from build123d import *

# Parameters (mm, degrees)
SKETCH1_R           = 250
SKETCH1_R_2         = 162.5
BOSS_EXTRUDE1_DEPTH = 9.5
SKETCH2_R           = 202.5
SKETCH2_R_2         = 192.5
CUT_EXTRUDE1_DEPTH  = 7


with BuildPart() as part:
    # Sketch1 → Boss-Extrude1 (new, symmetric)
    with BuildSketch(Plane(origin=(0, 0, 0), x_dir=(1, 0, 0), z_dir=(0, 1, 0))):
        with Locations(Location((0, 0, 0), (0, 0, 270))):
            Circle(SKETCH1_R)
        with Locations(Location((0, 0, 0), (0, 0, 270))):
            Circle(SKETCH1_R_2, mode=Mode.SUBTRACT)
    extrude(amount=BOSS_EXTRUDE1_DEPTH, both=True)

    # Sketch2 → Cut-Extrude1 (cut)
    with BuildSketch(Plane(origin=(0, 9.5, 0), x_dir=(1, 0, 0), z_dir=(0, 1, 0))):
        with Locations(Location((0, 0, 0), (0, 0, 270))):
            Circle(SKETCH2_R)
        with Locations(Location((0, 0, 0), (0, 0, 270))):
            Circle(SKETCH2_R_2, mode=Mode.SUBTRACT)
    extrude(amount=-CUT_EXTRUDE1_DEPTH, mode=Mode.SUBTRACT)


solid = part.part
CAD build for the part. Positions are in the model's coordinates, mm. A direction names the side the tool comes from. Round coordinates to 2 decimals unless told otherwise and drop trailing zeros. Order: outer loops, then holes, each group sorted by start corner. A loop starts at its lowest first (then second) coordinate and runs counter-clockwise, first axis right, second up. Notation, with made-up numbers: (89.5, 71) -> (108.5, 71) arc R11 ccw to (108.5, 89) -> close; hole circle Ø6 at (38, 66.5). An arc over 180 degrees is marked (long way). Write each question's results on one line, items separated by ' | '.
1. Cut at B-B (x = 0). Give the cut face in (y, z), plus the area to 4 significant figures.
Findings below:
outline: (-9.5, -250) -> (9.5, -250) -> (9.5, -202.5) -> (2.5, -202.5) -> (2.5, -192.5) -> (9.5, -192.5) -> (9.5, -162.5) -> (-9.5, -162.5) -> close; (-9.5, 162.5) -> (9.5, 162.5) -> (9.5, 192.5) -> (2.5, 192.5) -> (2.5, 202.5) -> (9.5, 202.5) -> (9.5, 250) -> (-9.5, 250) -> close | area: 3,185 mm²
2. 3-axis set-ups, long thin cutter, end or side, ignore diameter. For faces 1 (the face through (1, 9.5, 203)), 2 (the face through (-74, 2.5, 179)): which of +Z, -Z, +X, -X, +Y, -Y reach the whole face in a straight line?
Findings below:
face 1: +Z, -Z, +X, -X, +Y | face 2: +Y
3. Cut at D-D (x = 215.5). Give the cut face in (y, z).
Findings below:
outline: (-9.5, -126.73) -> (9.5, -126.73) -> (9.5, 126.73) -> (-9.5, 126.73) -> close
4. Pull direction X, two halves, no side cores. Call faces 3 (the face through (10.99, 0.13, -249.76)), 4 (the face through (137.02, -0.13, 87.36)), 5 (the face through (3, -9.5, 163)): pulls with the +X half, pulls with the -X half, needs draft (parallel to the pull), parting line crosses it, or undercut.
Findings below:
face 3: parting line crosses it | face 4: undercut | face 5: needs draft
5. Cut at A-A (z = 0). Give the cut face in (x, y), plus the area to 4 significant figures.
Findings below:
outline: (-250, -9.5) -> (-162.5, -9.5) -> (-162.5, 9.5) -> (-192.5, 9.5) -> (-192.5, 2.5) -> (-202.5, 2.5) -> (-202.5, 9.5) -> (-250, 9.5) -> close; (162.5, -9.5) -> (250, -9.5) -> (250, 9.5) -> (202.5, 9.5) -> (202.5, 2.5) -> (192.5, 2.5) -> (192.5, 9.5) -> (162.5, 9.5) -> close | area: 3,185 mm²
6. Flat gauge pins, fed straight in: P1, Ø10, axis at x = -33, y = -2, coming from the -Z side; P2, Ø1.5, axis at y = -5.5, z = 140, coming from the -X side; P3, Ø1.5, axis at x = -150, y = 3, coming from the -Z side. Where does each tip first touch, or does it go through?
Findings below:
P1: stops at z = -248.43 | P2: stops at x = -207.63 | P3: stops at z = -200.56
7. Cut at C-C (y = -6.5). Give the cut face in (x, z).
Findings below:
outline: circle Ø500 at (0, 0); hole circle Ø325 at (0, 0)
8. Wall check: line 1 along X through (y, z) = (-4, 0); line 2 along Z through (x, y) = (112.5, 4.5) (3 decimals); line 3 along X through (y, z) = (4, -44.5). Give the ranges that are in metal, low to high. Write a range as [from, to].
Findings below:
line 1: x = [-250, -162.5], [162.5, 250] | line 2: z = [-223.257, -168.375], [-156.205, -117.26], [117.26, 156.205], [168.375, 223.257] | line 3: x = [-246.01, -197.55], [-187.29, -156.29], [156.29, 187.29], [197.55, 246.01]
